Source: CAD feature listing. Evaluate the final solid. Frame: model axes, mm. Round coordinates to 2 decimals unless told otherwise and drop trailing zeros. Put each result on its own line as item: value. Start each with the question number.
1. Material intervals for L1, parallel to X at y = -3.2, z = -70.5; L2, parallel to X at y = -2.1, z = -0.5; L3, parallel to X at y = -1.25, z = -68, sorted ascending.
2. Cut plane A-A (z = -71). State how many separate pieces and enclosed holes the cut face has, then the cut area to 3 significant figures.
3. Contact query for flat-ended pins moving along their axis: pin 1 (2.5 mm diameter, centred on x = 21.5, y = -2, fed in from -Z); pin 2 (2 mm diameter, centred on y = -1.5, z = 39, fed in from -X); pin 3 (2.5 mm diameter, centred on x = 14.88, z = -33.5, fed in from -Y); pin 4 (2.5 mm diameter, centred on x = 3.5, y = -3.5, fed in from -Z). Output: stop coordinate, or through.
```python
from build123d import *

# Parameters (mm, degrees)
F0_R     = 1.95
F1_DEPTH = 5


with BuildPart() as f1:
    # F0 (on Front) → F1 (new body)
    with BuildSketch(Plane.XZ):
        with BuildLine():
            ThreePointArc((11.5969807084, 58.0333357261), (11.8982090371, 58.9962329808), (12, 60))
            ThreePointArc((12, 60), (10.5355339059, 63.5355339059), (7, 65))
            ThreePointArc((7, 65), (2.8266727082, 57.2462136402), (11.5969807084, 58.0333357261))
        make_face()
        with Locations((7, 60)):
            Circle(F0_R, mode=Mode.SUBTRACT)
        with BuildLine():
            ThreePointArc((11.5969807084, 58.0333357261), (2.8266727082, 57.2462136402), (7, 65))
            Line((7, 65), (0, 65))
            Line((0, 65), (-7, 65))
            ThreePointArc((-7, 65), (-3.4644660941, 63.5355339059), (-2, 60))
            ThreePointArc((-2, 60), (-5.9962329808, 55.1017909629), (-11.5969807084, 58.0333357261))
            add(Edge.make_bspline(
                [(-11.5969807084, 58.0333357261), (-8.259178384, 50.2313874739), (-5.7002681923, 15.299773588), (-20.5659226075, 6.5540384245), (-26.4394786751, 4.7883087979)],
                knots=[0, 0, 0, 0, 0.5815539161, 1, 1, 1, 1], degree=3))
            ThreePointArc((-26.4394786751, 4.7883087979), (-22.0164947943, 4.0123181189), (-20, 0))
            ThreePointArc((-20, 0), (-23.271638205, -4.69177637), (-28.8051062023, -3.2436348113))
            add(Edge.make_bspline(
                [(-28.8051062023, -3.2436348113), (-22.7247010924, -10.376554681), (-15.2262960098, -29.050287314), (-43.232798529, -73.227558015), (-58.8278773565, -81.4663794637)],
                knots=[0, 0, 0, 0, 0.3913654049, 1, 1, 1, 1], degree=3))
            Line((-58.8278773565, -81.4663794637), (-58.8278773565, -86.4663794637))
            Line((-58.8278773565, -86.4663794637), (-40.2264967561, -86.4663794637))
            add(Edge.make_bspline(
                [(-24.8, -81.4663794637), (-27.8363596976, -81.4270702004), (-35.2759175003, -83.0063000321), (-40.2264967561, -86.4663794637)],
                knots=[0, 0, 0, 0, 16.2165595046, 16.2165595046, 16.2165595046, 16.2165595046], degree=3))
            Line((-24.8, -81.4663794637), (-24.8, -66.4663794637))
            Line((-24.8, -66.4663794637), (-20, -66.4663794637))
            Line((-20, -66.4663794637), (-20, -81.4663794637))
            Line((-20, -81.4663794637), (0, -81.4663794637))
            Line((0, -81.4663794637), (20, -81.4663794637))
            Line((20, -81.4663794637), (20, -66.4663794637))
            Line((20, -66.4663794637), (24.8, -66.4663794637))
            Line((24.8, -66.4663794637), (24.8, -81.4663794637))
            add(Edge.make_bspline(
                [(24.8, -81.4663794637), (27.8363596976, -81.4270702004), (35.2759175003, -83.0063000321), (40.2264967561, -86.4663794637)],
                knots=[0, 0, 0, 0, 16.2165595046, 16.2165595046, 16.2165595046, 16.2165595046], degree=3))
            Line((40.2264967561, -86.4663794637), (58.8278773565, -86.4663794637))
            Line((58.8278773565, -86.4663794637), (58.8278773565, -81.4663794637))
            add(Edge.make_bspline(
                [(28.8051062023, -3.2436348113), (22.7247010924, -10.376554681), (15.2262960098, -29.050287314), (43.232798529, -73.227558015), (58.8278773565, -81.4663794637)],
                knots=[0, 0, 0, 0, 0.3913654049, 1, 1, 1, 1], degree=3))
            ThreePointArc((28.8051062023, -3.2436348113), (20.2037048496, -1.4126403755), (26.4394786751, 4.7883087979))
            add(Edge.make_bspline(
                [(11.5969807084, 58.0333357261), (8.259178384, 50.2313874739), (5.7002681923, 15.299773588), (20.5659226075, 6.5540384245), (26.4394786751, 4.7883087979)],
                knots=[0, 0, 0, 0, 0.5815539161, 1, 1, 1, 1], degree=3))
        make_face()
        with Locations((0, -66.8700714409)):
            Circle(F0_R, mode=Mode.SUBTRACT)
        with Locations((0, -46.8700714409)):
            Circle(F0_R, mode=Mode.SUBTRACT)
        with Locations((14.8781873236, -33.5044610186)):
            Circle(F0_R, mode=Mode.SUBTRACT)
        with BuildLine():
            add(Edge.make_bspline(
                [(0, 20.4110946506), (-2.5965298992, 8.6431102827), (-5.6864479557, 2.9892178718), (-12.2460462153, -2.4297779892)],
                knots=[0, 0, 0, 0, 25.9166184302, 25.9166184302, 25.9166184302, 25.9166184302], degree=3))
            add(Edge.make_bspline(
                [(0, 20.4110946506), (2.5965298992, 8.6431102827), (5.6864479557, 2.9892178718), (12.2460462153, -2.4297779892)],
                knots=[0, 0, 0, 0, 25.9166184302, 25.9166184302, 25.9166184302, 25.9166184302], degree=3))
            add(Edge.make_bspline(
                [(12.2460462153, -2.4297779892), (4.406365566, -11.6358492523), (7.9564843327, -24.7844345868), (0, -32.1476459503)],
                knots=[0, 0, 0, 0, 32.1421424934, 32.1421424934, 32.1421424934, 32.1421424934], degree=3))
            add(Edge.make_bspline(
                [(-12.2460462153, -2.4297779892), (-4.406365566, -11.6358492523), (-7.9564843327, -24.7844345868), (0, -32.1476459503)],
                knots=[0, 0, 0, 0, 32.1421424934, 32.1421424934, 32.1421424934, 32.1421424934], degree=3))
        make_face(mode=Mode.SUBTRACT)
        with BuildLine():
            ThreePointArc((30, 0), (29.0123181189, 2.9835052057), (26.4394786751, 4.7883087979))
            ThreePointArc((26.4394786751, 4.7883087979), (20.2037048496, -1.4126403755), (28.8051062023, -3.2436348113))
            ThreePointArc((28.8051062023, -3.2436348113), (29.69177637, -1.728361795), (30, 0))
        make_face()
        with Locations((25, 0)):
            Circle(F0_R, mode=Mode.SUBTRACT)
        with BuildLine():
            ThreePointArc((-2, 60), (-3.4644660941, 63.5355339059), (-7, 65))
            ThreePointArc((-7, 65), (-11.1733272918, 62.7537863598), (-11.5969807084, 58.0333357261))
            ThreePointArc((-11.5969807084, 58.0333357261), (-5.9962329808, 55.1017909629), (-2, 60))
        make_face()
        with Locations((-7, 60)):
            Circle(F0_R, mode=Mode.SUBTRACT)
        with BuildLine():
            ThreePointArc((-20, 0), (-22.0164947943, 4.0123181189), (-26.4394786751, 4.7883087979))
            ThreePointArc((-26.4394786751, 4.7883087979), (-29.7962951504, 1.4126403755), (-28.8051062023, -3.2436348113))
            ThreePointArc((-28.8051062023, -3.2436348113), (-23.271638205, -4.69177637), (-20, 0))
        make_face()
        with Locations((-25, 0)):
            Circle(F0_R, mode=Mode.SUBTRACT)
    extrude(amount=F1_DEPTH)


solid = f1.part
```
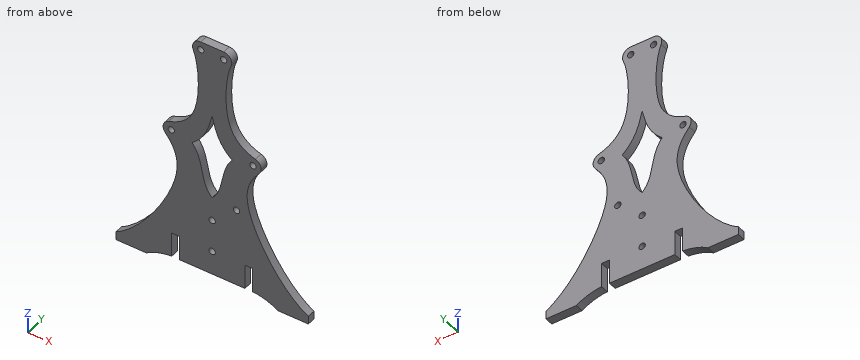
Solution:
1. L1: x = -45.45 to -24.8, -20 to 20, 24.8 to 45.45
1. L2: x = -29.97 to -26.88, -23.12 to -10.07, 10.07 to 23.12, 26.88 to 29.97
1. L3: x = -43.25 to -24.8, -20 to -1.59, 1.59 to 20, 24.8 to 43.25
2. separate pieces: 3
2. enclosed holes: 0
2. area: 411 mm^2
3. pin 1: stops at z = -66.47
3. pin 2: stops at x = -8.5
3. pin 3: passes through
3. pin 4: stops at z = -81.47
